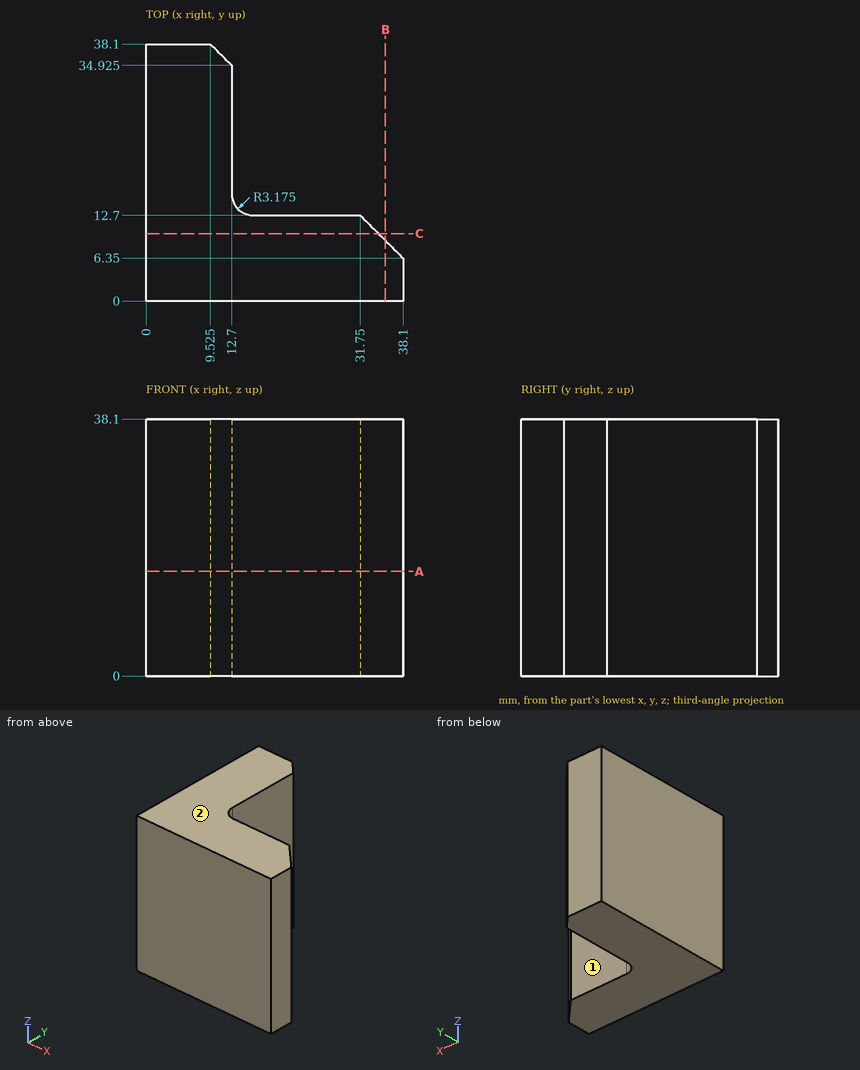
Input: dimensioned drawing with shaded views. Units: mm. Origin: part minimum x, y, z. A direction names the side the tool comes from. Coordinates: 2 decimals unless noted, no trailing zeros. Order: outer loops, then holes, each group sorted by start corner. A loop starts at its lowest first (then second) coordinate and runs counter-clockwise, first axis right, second up. Notation, with made-up numbers: (79.5, 5.25) - (136.5, 5.25) arc R18 cw to (136.5, 11.25) - close; hole circle Ø4 at (-33.5, 79). An arc over 180 degrees is marked (long way). Return JSON: item names as keys, results as strings. Group by question number.
1. Set-up query: the marked faces 1 and 2. Return all of +Z, -Z, +X, -X, +Y, -Y with unobstructed straight access to the full face (end or side cutting, diameter ignored); none if empty.
2. Pin query (flat end, axial travel): pin 1 (6 mm diameter, centred on y = 8, z = 10, fed in from -X); pin 2 (17.5 mm diameter, centred on x = 20.5, z = 14, fed in from +Y) (3 decimals); pin 3 (2 mm diameter, centred on y = 33, z = 6, fed in from +X). Return the tip coordinate at first contact, or that it passes through.
3. Cut plane A-A (z = 15.5). Output: boundary loops of the cut face in (x, y) (3 decimals).
4. Cut plane B-B (x = 35.5). Output: boundary loops of the cut face in (y, z), plus the area to 3 significant figures.
5. Cut plane C-C (y = 10). Output: boundary loops of the cut face in (x, z), plus the area to 3 significant figures.
6. Material intervals for line 1 along X through (y, z) = (33, 3); line 2 along X through (y, z) = (11.5, 26.5), sorted ascending. Write a range as [from, to].
Resolved:
{
 "1": {"face 1": "+Z, -Z, +X, +Y", "face 2": "+Z, +X, -X, +Y, -Y"},
 "2": {"pin 1": "stops at x = 0", "pin 2": "stops at y = 35.875", "pin 3": "stops at x = 12.7"},
 "3": {"outline": "(0, 0) - (38.1, 0) - (38.1, 6.35) - (31.75, 12.7) - (15.875, 12.7) arc R3.175 cw to (12.7, 15.875) - (12.7, 34.925) - (9.525, 38.1) - (0, 38.1) - close"},
 "4": {"outline": "(0, 0) - (8.95, 0) - (8.95, 38.1) - (0, 38.1) - close", "area": "341 mm²"},
 "5": {"outline": "(0, 0) - (34.45, 0) - (34.45, 38.1) - (0, 38.1) - close", "area": "1,310 mm²"},
 "6": {"line 1": "x = [0, 12.7]", "line 2": "x = [0, 32.95]"}
}
